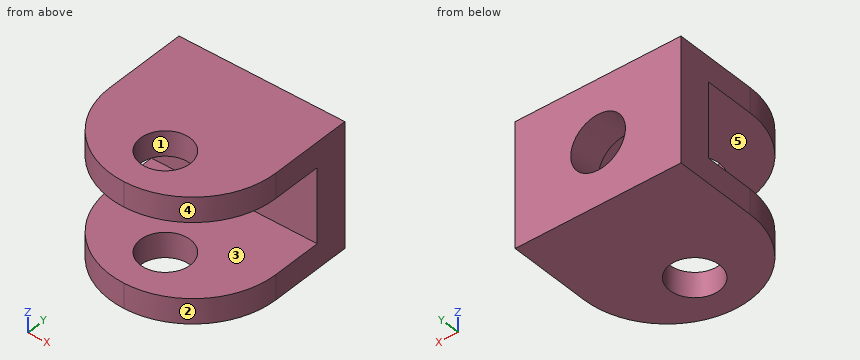
from build123d import *

# Parameters (mm, degrees)
SKETCH1_W                = 20
SKETCH1_H                = 15
BOSS_EXTRUDE1_DEPTH      = 4
SKETCH3_W                = 20
SKETCH3_H                = 3
BOSS_EXTRUDE2_DEPTH      = 16
M6_CLEARANCE_HOLE1_D     = 6.6
M6_CLEARANCE_HOLE1_DEPTH = 8
M6_CLEARANCE_HOLE1_TIP   = 1.982840043
SKETCH6_R                = 3
CUT_EXTRUDE1_DEPTH       = 15
FILLET1_R                = 10


with BuildPart() as part:
    # Sketch1 → Boss-Extrude1 (new body)
    with BuildSketch(Plane(origin=(0, 0, 0), x_dir=(1, 0, 0), z_dir=(0, 1, 0))):
        Rectangle(SKETCH1_W, SKETCH1_H)
    extrude(amount=BOSS_EXTRUDE1_DEPTH)

    # Sketch3 → Boss-Extrude2 (add)
    with BuildSketch(Plane.XZ):
        with Locations((0, -6)):
            Rectangle(SKETCH3_W, SKETCH3_H)
        with Locations((0, 6)):
            Rectangle(SKETCH3_W, SKETCH3_H)
    extrude(amount=BOSS_EXTRUDE2_DEPTH)

    # M6 Clearance Hole1
    with Locations(Plane.ZX.offset(4)):
        with Locations((0, 0)):
            Hole(M6_CLEARANCE_HOLE1_D / 2, depth=M6_CLEARANCE_HOLE1_DEPTH)
            with Locations((0, 0, -(M6_CLEARANCE_HOLE1_DEPTH + M6_CLEARANCE_HOLE1_TIP / 2))):  # 118° drill point
                Cone(0, M6_CLEARANCE_HOLE1_D / 2, M6_CLEARANCE_HOLE1_TIP, mode=Mode.SUBTRACT)

    # Sketch6 → Cut-Extrude1 (cut)
    with BuildSketch(Plane.XY.offset(-7.5)):
        with Locations((0, -10)):
            Circle(SKETCH6_R)
    extrude(amount=CUT_EXTRUDE1_DEPTH, mode=Mode.SUBTRACT)

    # Fillet1
    fillet1_edges = [part.edges().sort_by_distance(p)[0] for p in [
        (10, -16, -6),
        (10, -16, 6),
        (-10, -16, 6),
        (-10, -16, -6),
    ]]
    fillet(fillet1_edges, radius=FILLET1_R - 0.0001)  # a hair under: the kernel refuses the full size


solid = part.part
The listing builds one solid part. Answer for the finished solid, in the listing's coordinates (mm). Face numbers are marked on the shaded views. A direction names the side the tool comes from. Coordinates: 2 decimals unless noted, no trailing zeros. Order: outer loops, then holes, each group sorted by start corner. A loop starts at its lowest first (then second) coordinate and runs counter-clockwise, first axis right, second up.
Q1. Consider line 1 (Z direction, x = -7, y = -9); line 2 (Y direction, x = 0, z = 6.35); line 3 (Y direction, x = 3, z = -3.25). Determine where each line is inside the solid, lowest interval first.
Q2. A cutting plane is placed at B-B, the plane x = -1.75. Write down the section's boundary in (y, z), and give its area (3 significant figures).
Q3. For a pull along Y with two mould halves and no side action, classify the marked faces 1, 2 and 3 as pulls with the +Y half, pulls with the -Y half, needs draft (parallel to the pull), parting line crosses it, or undercut.
Q4. A cutting plane is placed at A-A, the plane z = 0. Write down the section's boundary in (x, y).
Q5. A cutting plane is placed at D-D, the plane y = 2.5. Write down the section's boundary in (x, z), and give its area (3 significant figures).
Q6. A cutting plane is placed at C-C, the plane y = -10.5. Write down the section's boundary in (x, z).
Q7. Which of the six approach directions +Z, -Z, +X, -X, +Y, -Y give full straight-line access (tool end or side, diameter ignored) to the marked faces 4 and 5?
Q8. Given P1, Ø4, axis at x = -2, y = -10, coming from the +Z side; P2, Ø1, axis at x = -7, y = -14, coming from the -Z side; P3, Ø2, axis at x = -7, z = 2.5, coming from the -Y side, each flat-ended and moving along its own axis, determine where each tip first touches the part or whether it passes through.
Answers follow:
1. line 1: z = -7.5 to -4.5, 4.5 to 7.5
1. line 2: y = -16 to -13, -7 to 4
1. line 3: y = 0 to 4
2. outline: (-15.85, -7.5) - (-12.44, -7.5) - (-12.44, -4.5) - (-15.85, -4.5) - close; (-15.85, 4.5) - (-12.44, 4.5) - (-12.44, 7.5) - (-15.85, 7.5) - close; (-7.56, -7.5) - (4, -7.5) - (4, -2.8) - (0, -2.8) - (0, -4.5) - (-7.56, -4.5) - close; (-7.56, 4.5) - (0, 4.5) - (0, 2.8) - (4, 2.8) - (4, 7.5) - (-7.56, 7.5) - close
2. area: 103 mm2
3. face 1: undercut
3. face 2: pulls with the -Y half
3. face 3: needs draft
4. outline: (-10, 0) - (-3.3, 0) - (-3.3, 4) - (-10, 4) - close; (3.3, 0) - (10, 0) - (10, 4) - (3.3, 4) - close
5. outline: (-10, -7.5) - (10, -7.5) - (10, 7.5) - (-10, 7.5) - close; hole circle Ø6.6 at (0, 0)
5. area: 266 mm2
6. outline: (-8.93, -7.5) - (-2.96, -7.5) - (-2.96, -4.5) - (-8.93, -4.5) - close; (-8.93, 4.5) - (-2.96, 4.5) - (-2.96, 7.5) - (-8.93, 7.5) - close; (2.96, -7.5) - (8.93, -7.5) - (8.93, -4.5) - (2.96, -4.5) - close; (2.96, 4.5) - (8.93, 4.5) - (8.93, 7.5) - (2.96, 7.5) - close
7. face 4: +Z, -Z, +X, -Y
7. face 5: +X, -X, -Y
8. P1: stops at z = 7.5
8. P2: passes through
8. P3: stops at y = 0
